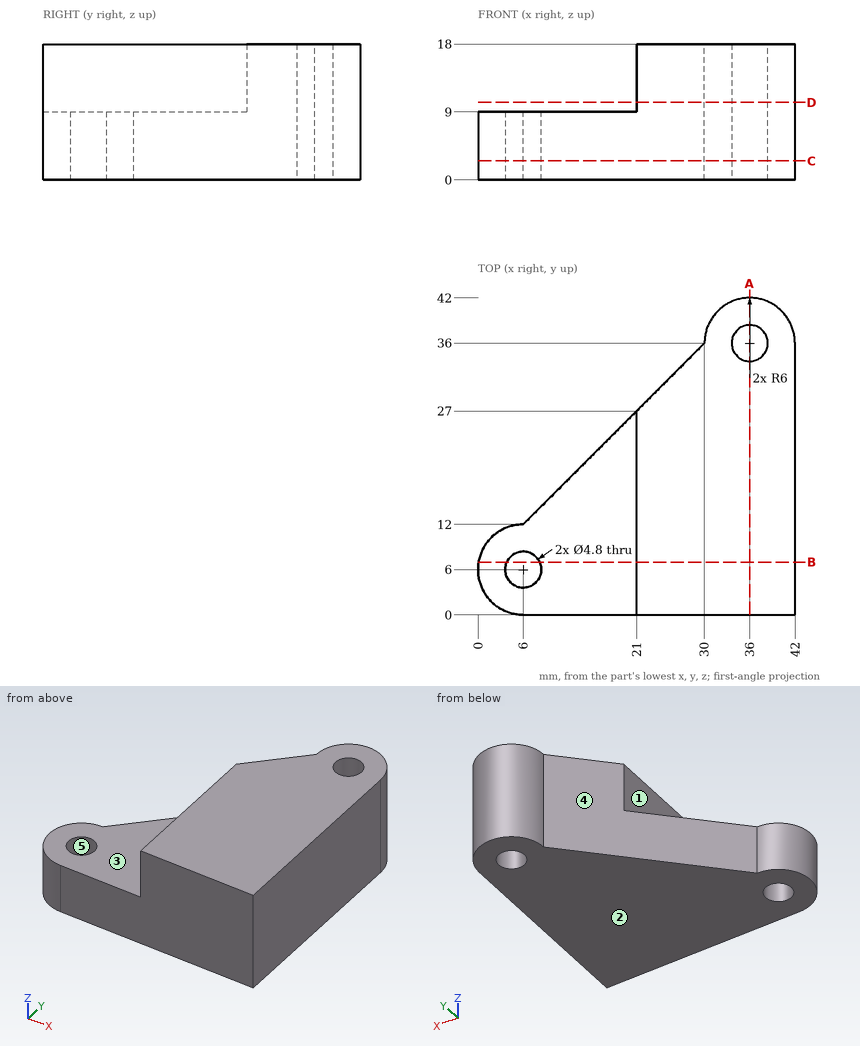
Study the drawing (mm; zero at the part's minimum x, y, z) and answer. A direction names the side the tool comes from. Coordinates: 2 decimals unless noted, no trailing zeros. Write each loop counter-clockwise with the first axis right and the second up, starting at its lowest first coordinate (ties: lowest second). Pieces come first, ordered by that corner, then holes. Notation, with made-up numbers: (-5, -22) - (31, -22) arc R12 ccw to (31, -8) - close; hole circle Ø2 at (-36.75, 61.25). An arc over 180 degrees is marked (long way). Put each result on its own line as item: value.
1. The part is cut by section A-A on x = 36. Give the vertices of the cut face in (y, z), plus the area to 3 significant figures.
Answer sheet:
outline: (0, 0) - (33.6, 0) - (33.6, 18) - (0, 18) - close; (38.4, 0) - (42, 0) - (42, 18) - (38.4, 18) - close
area: 670 mm^2
2. The part is cut by section C-C on z = 2.5. Give the vertices of the cut face in (x, y), plus the area to 3 significant figures.
Answer sheet:
outline: (6, 0) - (42, 0) - (42, 36) arc R6 ccw to (30, 36) - (6, 12) arc R6 ccw to start; hole circle Ø4.8 at (6, 6); hole circle Ø4.8 at (36, 36)
area: 1,080 mm^2
3. Find the intervals of material crossed by line 1 along Y through (x, z) = (6, 6.75); line 2 along Y through (x, z) = (36, 13); line 3 along X through (y, z) = (9, 16.5), in increasing order. Write a range as from..to.
Answer sheet:
line 1: y = 0..3.6, 8.4..12
line 2: y = 0..33.6, 38.4..42
line 3: x = 21..42
4. Flat-ended cylindrical pins translate along their axes: pin 1 Ø3 at (y, z) = (36.5, 12.5) entering from -X; pin 2 Ø3 at (x, z) = (14, 4.5) entering from +Y; pin 3 Ø8 at (y, z) = (26, 6.5) entering from -X. Find the tip coordinate at first contact, or state that the pin passes through.
Answer sheet:
pin 1: stops at x = 29
pin 2: stops at y = 21.5
pin 3: stops at x = 16
5. The part is cut by section D-D on z = 10.25. Give the vertices of the cut face in (x, y), plus the area to 3 significant figures.
Answer sheet:
outline: (21, 0) - (42, 0) - (42, 36) arc R6 ccw to (30, 36) - (21, 27) - close; hole circle Ø4.8 at (36, 36)
area: 754 mm^2
6. The part is cut by section B-B on y = 7. Give the vertices of the cut face in (x, z), plus the area to 3 significant figures.
Answer sheet:
outline: (0.08, 0) - (3.82, 0) - (3.82, 9) - (0.08, 9) - close; (8.18, 0) - (42, 0) - (42, 18) - (21, 18) - (21, 9) - (8.18, 9) - close
area: 527 mm^2
7. A tool of negligible diameter and unlimited length cuts with its end or side. For the marked faces 1 and 2, from which of +Z, -Z, +X, -X, +Y, -Y can it reach the whole face along a straight path? Write none if from no direction.
Answer sheet:
face 1: +Z, -X, +Y, -Y
face 2: -Z, +X, -X, +Y, -Y
8. Determine the mould class of the marked faces 3, 4 and 5 for opening direction Y: pulls with the +Y half, pulls with the -Y half, needs draft (parallel to the pull), parting line crosses it, or undercut.
Answer sheet:
face 3: needs draft
face 4: pulls with the +Y half
face 5: undercut
